Part model, mm, in its own coordinate system. A direction names the side the tool comes from. Round coordinates to 2 decimals unless told otherwise and drop trailing zeros. Loops run counter-clockwise (first coordinate to the right, second up) from the corner with the lowest first, then second, coordinate; pieces in that order, holes last. Notation, with made-up numbers: M -5,55 L 47,55 A15 ccw 47,84 Z; hole C 71.5,82.5 d7. An arc over 180 degrees is marked long. Put each result on its own line as item: value. Start each with the question number.
1) Slice it at B-B on y = 6. Give the cut face in (x, z), then the cut area to 3 significant figures.
2) Pull direction X, two halves, no side cores. Call faces 1 (the flat face through (-36.472, 16, -2)), 2 (the flat face through (-10.716, 19.214, -1.027)), 3 (the flat face through (-2, 6, -1.921)): +X half, -X half, draft (parallel to the pull), parting line (faces both ways), or undercut.
3) Drop flat-ended pins along their axis: pin 1 Ø4 at (x, y) = (0.5, 5) entering from +Z; pin 2 Ø2.5 at (y, z) = (7, 0) entering from -X; pin 3 Ø3 at (x, z) = (-30.5, -0.5) entering from +Y. Give the stop position or say it passes through.
4) Slice it at C-C on x = -10. Give the cut face in (y, z), then the cut area to 3 significant figures.
5) Which spindle directions (+Z, -Z, +X, -X, +Y, -Y) get a long thin tool onto all of the face, cutting with end or side? Do faces 4 (the flat face through (-14.328, 6, 0)), 5 (the flat face through (-2, 12.7, 0)), 6 (the flat face through (-2, 15, 1.213)). Say none if no direction does.
6) Probe line 1 along X through (y, z) = (1, 4.25); line 2 along Z through (x, y) = (2.5, 16.25); line 3 along X through (y, z) = (6.25, -4). List the from-to ranges inside material, lowest first.
7) Slice it at A-A on z = 2. Give the cut face in (x, y), then the cut area to 3 significant figures.
8) Slice it at D-D on z = -0.5. Give the cut face in (x, y).
```python
from build123d import *

# Parameters (mm, degrees)
F0_W     = 28.655802
F0_H     = 8.69454
F1_DEPTH = 12.7
F2_W     = 22.303285
F2_H     = 6.268458
F3_DEPTH = 50.8
F5_DEPTH = 50.8
F6_W     = 22.303285
F6_H     = 3.134229
F7_DEPTH = 25.4


with BuildPart() as f1:
    # F0 (on Front) → F1 (new body)
    with BuildSketch(Plane.XZ):
        Rectangle(F0_W, F0_H)
    extrude(amount=-F1_DEPTH)

    # F2 (on face) → F3 (cut)
    with BuildSketch(Plane.XZ):
        with Locations((-2.270672, 1.213041)):
            Rectangle(F2_W, F2_H)
    extrude(amount=-F3_DEPTH, mode=Mode.SUBTRACT)

    # F4 (on face) → F5 (join)
    with BuildSketch(Plane.YZ.offset(14.327901)):
        Polygon((12.7, 4.34727), (12.7, -4.34727), (23.239153, -4.34727), align=None)
    extrude(amount=-F5_DEPTH)

    # F6 (on face) → F7 (cut)
    with BuildSketch(Plane.XZ.offset(-12.7)):
        with Locations((-2.270672, 2.780156)):
            Rectangle(F6_W, F6_H)
    extrude(amount=-F7_DEPTH, mode=Mode.SUBTRACT)


solid = f1.part
```
Recorded:
1. outline: M -14.33,-4.35 L 14.33,-4.35 L 14.33,4.35 L 8.88,4.35 L 8.88,-1.92 L -13.42,-1.92 L -13.42,4.35 L -14.33,4.35 Z
1. area: 109 mm2
2. face 1: -X half
2. face 2: draft
2. face 3: undercut
3. pin 1: stops at z = -1.92
3. pin 2: stops at x = -14.33
3. pin 3: stops at y = 20.39
4. outline: M 0,-4.35 L 23.24,-4.35 L 16.5,1.21 L 12.7,1.21 L 12.7,-1.92 L 0,-1.92 Z
4. area: 70.7 mm2
5. face 4: +Z, -Z, -X, -Y
5. face 5: +Z, -Y
5. face 6: +Z, +Y, -Y
6. line 1: x = -14.33 to -13.42, 8.88 to 14.33
6. line 2: z = -4.35 to 1.21
6. line 3: x = -14.33 to 14.33
7. outline: M -36.47,12.7 L -14.33,12.7 L -14.33,0 L -13.42,0 L -13.42,15.55 L -36.47,15.55 Z; M 8.88,0 L 14.33,0 L 14.33,15.55 L 8.88,15.55 Z
7. area: 162 mm2
8. outline: M -36.47,12.7 L -14.33,12.7 L -14.33,0 L -13.42,0 L -13.42,12.7 L 8.88,12.7 L 8.88,0 L 14.33,0 L 14.33,18.58 L -36.47,18.58 Z
